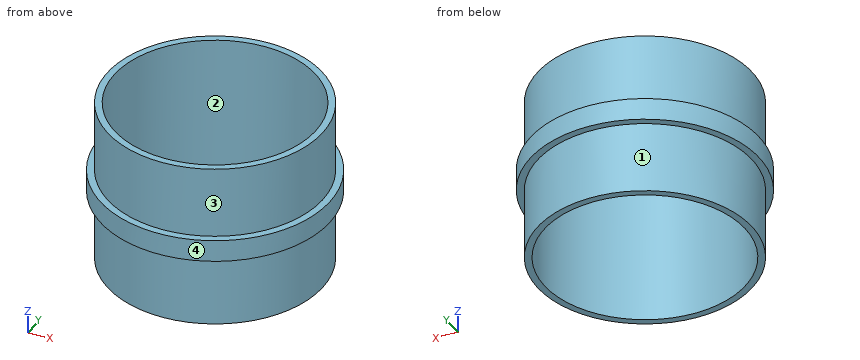
```python
from build123d import *

# Parameters (mm, degrees)
F0_R     = 9.75
F0_R_2   = 9.125
F1_DEPTH = 7.5
F2_R     = 10.398155
F2_R_2   = 9.75
F3_DEPTH = 1


with BuildPart() as f1:
    # F0 (on Top) → F1 (new body, symmetric)
    with BuildSketch(Plane.XY):
        Circle(F0_R)
        Circle(F0_R_2, mode=Mode.SUBTRACT)
    extrude(amount=F1_DEPTH, both=True)

    # F2 (on Top) → F3 (join, symmetric)
    with BuildSketch(Plane.XY):
        Circle(F2_R)
        Circle(F2_R_2, mode=Mode.SUBTRACT)
    extrude(amount=F3_DEPTH, both=True)


solid = f1.part
```
Input: part model. Units: mm. Frame: model coordinates. Face numbers are marked on the shaded views. A direction names the side the tool comes from. Give positions to 0.01 mm unless a question says otherwise; leave off trailing zeros. Loops run counter-clockwise (first coordinate to the right, second up) from the corner with the lowest first, then second, coordinate; pieces in that order, holes last.
1) Section query A-A on y = 0. Return the cut outline in (x, z) (3 decimals).
A:
outline: (-10.398, -1) - (-9.75, -1) - (-9.75, -7.5) - (-9.125, -7.5) - (-9.125, 7.5) - (-9.75, 7.5) - (-9.75, 1) - (-10.398, 1) - close; (9.125, -7.5) - (9.75, -7.5) - (9.75, -1) - (10.398, -1) - (10.398, 1) - (9.75, 1) - (9.75, 7.5) - (9.125, 7.5) - close
2) Contact query for flat-ended pins moving along their axis: pin 1 (10.5 mm diameter, centred on x = 0, y = -2, fed in from -Z); pin 2 (4 mm diameter, centred on x = -8, z = -4.5, fed in from -Y); pin 3 (3 mm diameter, centred on y = -7, z = 1.5, fed in from -X); pin 4 (1 mm diameter, centred on y = 5, z = 6, fed in from -X). Output: stop coordinate, or through.
A:
pin 1: passes through
pin 2: stops at y = -7.69
pin 3: stops at x = -8.77
pin 4: stops at x = -8.65
3) Section query C-C on z = 1.5. Return the cut outline in (x, y) (3 decimals), and give its area (3 significant figures).
A:
outline: circle Ø19.5 at (0, 0); hole circle Ø18.25 at (0, 0)
area: 37.1 mm2
4) Line query: L1, parallel to Y at x = 0, z = 1.5 (3 decimals); L2, parallel to Z at x = -9.25, y = 3.5; L3, parallel to Y at x = -2, z = -5.5. Output: solid intervals per line, ascending.
A:
L1: y = -9.75 to -9.125, 9.125 to 9.75
L2: z = -1 to 1
L3: y = -9.54 to -8.9, 8.9 to 9.54
5) Mould query, pull axis Y, two halves, no side actions, for the marked faces 1 and 2. Classes: released by +Y, released by -Y, zero draft, split by the parting line, or undercut.
A:
face 1: split by the parting line
face 2: undercut
6) Reachability of the marked faces 3 and 4 from +Z, -Z, +X, -X, +Y, -Y: full face, straight path, thin tool, end or side. Return the list, or none.
A:
face 3: +Z
face 4: +Z, -Z
